Geometry check sheet. Reference: the model listing, model coordinates, mm. A direction names the side the tool comes from. Round coordinates to 2 decimals unless told otherwise and drop trailing zeros. Loops run counter-clockwise (first coordinate to the right, second up) from the corner with the lowest first, then second, coordinate; pieces in that order, holes last.
```python
from build123d import *

# Parameters (mm, degrees)
ESQUISSE1_W              = 70
ESQUISSE1_H              = 70
BOSS_EXTRU_4_DEPTH       = 30
ESQUISSE5_W              = 60
ESQUISSE5_H              = 60
ENL_V_MAT_EXTRU_3_DEPTH  = 23
ESQUISSE6_R              = 5
ENL_V_MAT_EXTRU_4_DEPTH  = 23
ESQUISSE28_W             = 10
ESQUISSE28_H             = 30
BOSS_EXTRU_8_DEPTH       = 5
BOSS_EXTRU_9_DEPTH       = 10
ESQUISSE30_W             = 10
ESQUISSE30_H             = 30
BOSS_EXTRU_10_DEPTH      = 5
BOSS_EXTRU_14_DEPTH      = 10
ENL_V_MAT_EXTRU_6_DEPTH  = 10
ENL_V_MAT_EXTRU_15_DEPTH = 14


with BuildPart() as part:
    # Esquisse1 → Boss.-Extru.4 (new body)
    with BuildSketch(Plane(origin=(0, 0, 0), x_dir=(1, 0, 0), z_dir=(0, 1, 0))):
        with Locations((35, 35)):
            Rectangle(ESQUISSE1_W, ESQUISSE1_H)
    extrude(amount=BOSS_EXTRU_4_DEPTH)

    # Esquisse5 → Enlèv. mat.-Extru.3 (cut)
    with BuildSketch(Plane(origin=(0, 0, 0), x_dir=(-1, 0, 0), z_dir=(0, -1, 0))):
        with Locations((-35, 35)):
            Rectangle(ESQUISSE5_W, ESQUISSE5_H)
    extrude(amount=-ENL_V_MAT_EXTRU_3_DEPTH, mode=Mode.SUBTRACT)

    # Esquisse6 → Enlèv. mat.-Extru.4 (cut)
    with BuildSketch(Plane(origin=(0, 23, 0), x_dir=(-1, 0, 0), z_dir=(0, -1, 0))):
        with Locations(Location((-35, 35, 0), (0, 0, 90))):
            Circle(ESQUISSE6_R)
    extrude(amount=-ENL_V_MAT_EXTRU_4_DEPTH, mode=Mode.SUBTRACT)

    # Esquisse28 → Boss.-Extru.8 (add, symmetric)
    with BuildSketch(Plane.XZ):
        with Locations((55.004966989, -85)):
            Rectangle(ESQUISSE28_W, ESQUISSE28_H)
    extrude(amount=BOSS_EXTRU_8_DEPTH, both=True)

    # Esquisse29 → Boss.-Extru.9 (add)
    with BuildSketch(Plane(origin=(60.004966989, 0, 0), x_dir=(0, 0, -1), z_dir=(1, 0, 0))):
        Polygon((98.641624501, -8.437704854), (100, -5), (85, -5), (97.962436751, -10.156557281), align=None)
    extrude(amount=-BOSS_EXTRU_9_DEPTH)

    # Esquisse30 → Boss.-Extru.10 (add, symmetric)
    with BuildSketch(Plane.XZ):
        with Locations((15.004966989, -85)):
            Rectangle(ESQUISSE30_W, ESQUISSE30_H)
    extrude(amount=BOSS_EXTRU_10_DEPTH, both=True)

    # Esquisse39 → Boss.-Extru.14 (add)
    with BuildSketch(Plane.ZY.offset(-10.004966989)):
        Polygon((-100, -5), (-95.960946885, -15.231620103), (-85, -5), align=None)
    extrude(amount=-BOSS_EXTRU_14_DEPTH)

    # Esquisse40 → Enlèv. mat.-Extru.6 (cut)
    with BuildSketch(Plane(origin=(0, -34.827896321, -88.22508495), x_dir=(-1, 0, 0), z_dir=(0, -0.3671866467775486, -0.930147282116257))):
        Polygon((-20.004966989, 21.067928267), (-20.004966989, 22.067928267), (-10.004966989, 21.067928267), align=None)
    extrude(amount=-ENL_V_MAT_EXTRU_6_DEPTH, mode=Mode.SUBTRACT)

    # Esquisse41 → Enlèv. mat.-Extru.15 (cut)
    with BuildSketch(Plane(origin=(0, -34.85291455, -88.203912367), x_dir=(-1, 0, 0), z_dir=(0, -0.36749110102927884, -0.9300270375985252))):
        Polygon((-60.004966989, 27.554450861), (-60.004966989, 26.554450861), (-50.004966989, 26.554450861), align=None)
    extrude(amount=-ENL_V_MAT_EXTRU_15_DEPTH, mode=Mode.SUBTRACT)


solid = part.part
```
1) Sectioned sample at B-B, the plane y = 15. Record the cut outline in (x, z).
Report:
outline: (0, -70) - (70, -70) - (70, 0) - (0, 0) - close; hole (5, -65) - (65, -65) - (65, -5) - (5, -5) - close
2) Scan lines: line 1 along X through (y, z) = (19, -62); line 2 along X through (y, z) = (24, -35); line 3 along Z through (x, y) = (25, 1.5). Record each from-to range of solid material in increasing order.
Report:
line 1: x = 0 to 5, 65 to 70
line 2: x = 0 to 30, 40 to 70
line 3: z = -70 to -65, -5 to 0
3) Access from +Z, -Z, +X, -X, +Y, -Y to the whole of each face (thin tool, end or side, straight path). Record for faces 1 (the face through (5, 11, -35)), 2 (the face through (20.005, -2, -85)), 3 (the face through (55, -3, -70)).
Report:
face 1: -Y
face 2: -Z, +Y, -Y
face 3: +Z, +X, -X, -Y
4) Sectioned sample at D-D, the plane x = 22. Record the cut outline in (y, z), then the cut area to 3 significant figures.
Report:
outline: (0, -70) - (30, -70) - (30, 0) - (0, 0) - (0, -5) - (23, -5) - (23, -65) - (0, -65) - close
area: 720 mm2
5) Sectioned sample at C-C, the plane x = 35. Record the cut outline in (y, z).
Report:
outline: (0, -70) - (30, -70) - (30, -40) - (23, -40) - (23, -65) - (0, -65) - close; (0, -5) - (23, -5) - (23, -30) - (30, -30) - (30, 0) - (0, 0) - close
6) Gauge pin test, flat ends, axial feed: pin 1 (11.5 mm diameter, centred on x = 44.5, y = 13.5, fed in from -Z); pin 2 (2 mm diameter, centred on x = 13, z = -64.5, fed in from -Y); pin 3 (4.5 mm diameter, centred on y = 0.5, z = -92, fed in from -X); pin 4 (6 mm diameter, centred on x = 35, z = -35, fed in from +Y). Record the tip position at first contact, or that the pin passes through.
Report:
pin 1: stops at z = -70
pin 2: stops at y = 0
pin 3: stops at x = 10
pin 4: passes through
7) Mould release check, pull along Z, two halves, no side actions. Record for faces 4 (the face through (14.93, -10.04, -98.01)), 5 (the face through (35, 15, 0)), 6 (the face through (35, 11, -5)), 7 (the face through (70, 15, -35)): +Z half, -Z half, draft (parallel to the pull), parting line (faces both ways), or undercut.
Report:
face 4: -Z half
face 5: +Z half
face 6: undercut
face 7: draft
8) Sectioned sample at A-A, the plane z = -35. Record the cut outline in (x, y).
Report:
outline: (0, 0) - (5, 0) - (5, 23) - (30, 23) - (30, 30) - (0, 30) - close; (40, 23) - (65, 23) - (65, 0) - (70, 0) - (70, 30) - (40, 30) - close
